from build123d import *

# Parameters (mm, degrees)
ESQUISSE1_R                  = 23.35
BOSS_EXTRU_1_DEPTH           = 5
ESQUISSE2_W                  = 37
ESQUISSE2_H                  = 8
ESQUISSE2_W_2                = 33.6
ESQUISSE2_H_2                = 14.6
ENL_V_MAT_EXTRU_4_DEPTH      = 3
ESQUISSE10_R                 = 23.35
BOSS_EXTRU_2_DEPTH           = 60
ENL_V_MAT_EXTRU_5_DEPTH      = 73.90709842
ENL_V_MAT_EXTRU_5_DEPTH_BACK = 73.90709842
ESQUISSE11_W                 = 20
ESQUISSE11_H                 = 45
ENL_V_MAT_EXTRU_6_DEPTH      = 73.90709842
ENL_V_MAT_EXTRU_6_DEPTH_BACK = 73.90709842
ESQUISSE12_W                 = 20
ESQUISSE12_H                 = 45
ESQUISSE13_W                 = 18.2
ESQUISSE13_H                 = 4.5
ESQUISSE13_W_2               = 16.2
ESQUISSE13_H_2               = 2.5
BOSS_EXTRU_4_DEPTH           = 50
ENL_V_MAT_EXTRU_7_DEPTH      = 65.151734193
ENL_V_MAT_EXTRU_7_DEPTH_BACK = 17
ESQUISSE16_W                 = 15
ESQUISSE16_H                 = 5
BOSS_EXTRU_5_DEPTH           = 20
BOSS_EXTRU_6_DEPTH           = 15
BOSS_EXTRU_7_START           = -5
ESQUISSE18_R                 = 1.5
BOSS_EXTRU_7_DEPTH           = 5
BOSS_EXTRU_8_DEPTH           = 12
BOSS_EXTRU_9_DEPTH           = 23


with BuildPart() as part:
    # Esquisse1 → Boss.-Extru.1 (new body)
    with BuildSketch(Plane(origin=(0, 0, 0), x_dir=(1, 0, 0), z_dir=(0, 1, 0))):
        with Locations(Location((0, 0, 0), (0, 0, 270))):
            Circle(ESQUISSE1_R)
    extrude(amount=BOSS_EXTRU_1_DEPTH)

    # Esquisse2 → Enlèv. mat.-Extru.4 (cut)
    with BuildSketch(Plane(origin=(0, 5, 0), x_dir=(1, 0, 0), z_dir=(0, 1, 0))):
        with Locations((0, 6)):
            Rectangle(ESQUISSE2_W, ESQUISSE2_H)
        with Locations((0, -6.3)):
            Rectangle(ESQUISSE2_W_2, ESQUISSE2_H_2)
    extrude(amount=-ENL_V_MAT_EXTRU_4_DEPTH, mode=Mode.SUBTRACT)

    # Esquisse10 → Boss.-Extru.2 (add)
    with BuildSketch(Plane(origin=(0, 5, 0), x_dir=(1, 0, 0), z_dir=(0, 1, 0))):
        with Locations(Location((0, 0, 0), (0, 0, 270))):
            Circle(ESQUISSE10_R)
        with BuildLine():
            ThreePointArc((-16.8, -13.175071157), (-6.969307713, 20.180467041), (21.35, 0))
            ThreePointArc((21.35, 0), (20.180467041, -6.969307713), (16.8, -13.175071157))
            Line((16.8, -13.175071157), (16.8, -13.6))
            Line((16.8, -13.6), (16.457900838, -13.6))
            ThreePointArc((16.457900838, -13.6), (0, -21.35), (-16.457900838, -13.6))
            Line((-16.457900838, -13.6), (-16.8, -13.6))
            Line((-16.8, -13.6), (-16.8, -13.175071157))
        make_face(mode=Mode.SUBTRACT)
    extrude(amount=BOSS_EXTRU_2_DEPTH)

    # Esquisse11 → Enlèv. mat.-Extru.5 (cut, two sides: drawn at the far end of the back side and taken through both)
    with BuildSketch(Plane.XY.offset(-ENL_V_MAT_EXTRU_5_DEPTH_BACK)):
        with Locations((0, 27.5)):
            Rectangle(ESQUISSE11_W, ESQUISSE11_H)
    extrude(amount=ENL_V_MAT_EXTRU_5_DEPTH + ENL_V_MAT_EXTRU_5_DEPTH_BACK, mode=Mode.SUBTRACT)

    # Esquisse12 → Enlèv. mat.-Extru.6 (cut, two sides: drawn at the far end of the back side and taken through both)
    with BuildSketch(Plane(origin=(0, 0, 0), x_dir=(0, 0, -1), z_dir=(1, 0, 0)).offset(-ENL_V_MAT_EXTRU_6_DEPTH_BACK)):
        with Locations((0, 27.5)):
            Rectangle(ESQUISSE12_W, ESQUISSE12_H)
    extrude(amount=ENL_V_MAT_EXTRU_6_DEPTH + ENL_V_MAT_EXTRU_6_DEPTH_BACK, mode=Mode.SUBTRACT)

    # Esquisse13 → Boss.-Extru.4 (add)
    # profile 1 of 3: a face of its own
    with BuildSketch(Plane(origin=(0, 5, 0), x_dir=(1, 0, 0), z_dir=(0, 1, 0))):
        with BuildLine():
            Line((17.8, 2), (-17.8, 2))
            Line((-17.8, 2), (-17.8, -11.789083934))
            ThreePointArc((-17.8, -11.789083934), (-17.31387421, -12.49208789), (-16.8, -13.175071157))
            Line((-16.8, -13.175071157), (-16.8, 1))
            Line((-16.8, 1), (16.8, 1))
            Line((16.8, 1), (16.8, -13.175071157))
            ThreePointArc((16.8, -13.175071157), (17.31387421, -12.49208789), (17.8, -11.789083934))
            Line((17.8, -11.789083934), (17.8, 2))
        make_face()
    # profile 2 of 3: a face of its own
    with BuildSketch(Plane(origin=(0, 5, 0), x_dir=(1, 0, 0), z_dir=(0, 1, 0))):
        with Locations((0, -15.85)):
            Rectangle(ESQUISSE13_W, ESQUISSE13_H)
        with Locations((0, -15.85)):
            Rectangle(ESQUISSE13_W_2, ESQUISSE13_H_2, mode=Mode.SUBTRACT)
    # profile 3 of 3: a face of its own
    with BuildSketch(Plane(origin=(0, 5, 0), x_dir=(1, 0, 0), z_dir=(0, 1, 0))):
        with Locations((0, -15.85)):
            Rectangle(ESQUISSE13_W_2, ESQUISSE13_H_2)
    extrude(amount=BOSS_EXTRU_4_DEPTH)

    # Esquisse15 → Enlèv. mat.-Extru.7 (cut, two sides: drawn at the far end of the back side and taken through both)
    with BuildSketch(Plane(origin=(0, 55, 0), x_dir=(1, 0, 0), z_dir=(0, 1, 0)).offset(-ENL_V_MAT_EXTRU_7_DEPTH_BACK)):
        Polygon((8.1, -14.6), (-8.1, -14.6), (-8.1, -17.1), (-6.1, -17.1), (-6.1, -18.1), (6.1, -18.1), (6.1, -17.1), (8.1, -17.1), align=None)
    extrude(amount=ENL_V_MAT_EXTRU_7_DEPTH + ENL_V_MAT_EXTRU_7_DEPTH_BACK, mode=Mode.SUBTRACT)

    # Esquisse16 → Boss.-Extru.5 (add)
    with BuildSketch(Plane(origin=(0, 5, 0), x_dir=(1, 0, 0), z_dir=(0, 1, 0))):
        with Locations((0, 15.5)):
            Rectangle(ESQUISSE16_W, ESQUISSE16_H)
    extrude(amount=BOSS_EXTRU_5_DEPTH)

    # Esquisse17 → Boss.-Extru.6 (add)
    with BuildSketch(Plane(origin=(0, 25, 0), x_dir=(1, 0, 0), z_dir=(0, 1, 0))):
        Polygon((7.5, 18), (-0.6, 18), (-0.6, 17), (5.6, 17), (5.6, 14), (-5.6, 14), (-5.6, 16.758406292), (-5.6, 18), (-7.5, 18), (-7.5, 13), (7.5, 13), align=None)
    extrude(amount=BOSS_EXTRU_6_DEPTH)

    # Esquisse18 → Boss.-Extru.7 (add)
    # profile 1 of 4: a face of its own
    with BuildSketch(Plane(origin=(0, 65, 0), x_dir=(1, 0, 0), z_dir=(0, 1, 0)).offset(BOSS_EXTRU_7_START)):
        with BuildLine():
            Line((-11.385882097, 13.385882097), (-11.385882097, 20.385882097))
            ThreePointArc((-11.385882097, 20.385882097), (-16.510943341, 16.510943341), (-20.385882097, 11.385882097))
            Line((-20.385882097, 11.385882097), (-13.385882097, 11.385882097))
            ThreePointArc((-13.385882097, 11.385882097), (-11.971668535, 11.971668535), (-11.385882097, 13.385882097))
        make_face()
        with Locations(Location((-13.385882097, 13.385882097, 0), (0, 0, 270))):
            Circle(ESQUISSE18_R, mode=Mode.SUBTRACT)
    # profile 2 of 4: a face of its own
    with BuildSketch(Plane(origin=(0, 65, 0), x_dir=(1, 0, 0), z_dir=(0, 1, 0)).offset(BOSS_EXTRU_7_START)):
        with BuildLine():
            ThreePointArc((20.385882097, 11.385882097), (16.510943341, 16.510943341), (11.385882097, 20.385882097))
            Line((11.385882097, 20.385882097), (11.385882097, 13.385882097))
            ThreePointArc((11.385882097, 13.385882097), (11.971668535, 11.971668535), (13.385882097, 11.385882097))
            Line((13.385882097, 11.385882097), (20.385882097, 11.385882097))
        make_face()
        with Locations(Location((13.385882097, 13.385882097, 0), (0, 0, 270))):
            Circle(ESQUISSE18_R, mode=Mode.SUBTRACT)
    # profile 3 of 4: a face of its own
    with BuildSketch(Plane(origin=(0, 65, 0), x_dir=(1, 0, 0), z_dir=(0, 1, 0)).offset(BOSS_EXTRU_7_START)):
        with BuildLine():
            Line((-13.385882097, -11.385882097), (-20.385882097, -11.385882097))
            ThreePointArc((-20.385882097, -11.385882097), (-16.510943341, -16.510943341), (-11.385882097, -20.385882097))
            Line((-11.385882097, -20.385882097), (-11.385882097, -13.385882097))
            ThreePointArc((-11.385882097, -13.385882097), (-11.971668535, -11.971668535), (-13.385882097, -11.385882097))
        make_face()
        with Locations(Location((-13.385882097, -13.385882097, 0), (0, 0, 270))):
            Circle(ESQUISSE18_R, mode=Mode.SUBTRACT)
    # profile 4 of 4: a face of its own
    with BuildSketch(Plane(origin=(0, 65, 0), x_dir=(1, 0, 0), z_dir=(0, 1, 0)).offset(BOSS_EXTRU_7_START)):
        with BuildLine():
            ThreePointArc((11.385882097, -20.385882097), (16.510943341, -16.510943341), (20.385882097, -11.385882097))
            Line((20.385882097, -11.385882097), (13.385882097, -11.385882097))
            ThreePointArc((13.385882097, -11.385882097), (11.971668535, -11.971668535), (11.385882097, -13.385882097))
            Line((11.385882097, -13.385882097), (11.385882097, -20.385882097))
        make_face()
        with Locations(Location((13.385882097, -13.385882097, 0), (0, 0, 270))):
            Circle(ESQUISSE18_R, mode=Mode.SUBTRACT)
    extrude(amount=BOSS_EXTRU_7_DEPTH)

    # Esquisse33 → Boss.-Extru.8 (add)
    with BuildSketch(Plane(origin=(0, 5, 0), x_dir=(1, 0, 0), z_dir=(0, 1, 0))):
        with BuildLine():
            Line((-19.5, 2), (-18.5, 2))
            Line((-18.5, 2), (-18.5, 10))
            Line((-18.5, 10), (18.5, 10))
            Line((18.5, 10), (18.5, 2))
            Line((18.5, 2), (19.5, 2))
            Line((19.5, 2), (19.5, 8.693244504))
            Line((19.5, 8.693244504), (19.5, 10))
            Line((19.5, 10), (18.863257937, 10))
            ThreePointArc((18.863257937, 10), (18.587432982, 10.503800986), (18.298155645, 11))
            Line((18.298155645, 11), (18.128988944, 11))
            Line((18.128988944, 11), (-18.298155645, 11))
            ThreePointArc((-18.298155645, 11), (-18.587432982, 10.503800986), (-18.863257937, 10))
            Line((-18.863257937, 10), (-19.5, 10))
            Line((-19.5, 10), (-19.5, 8.693244504))
            Line((-19.5, 8.693244504), (-19.5, 2))
        make_face()
    extrude(amount=BOSS_EXTRU_8_DEPTH)

    # Esquisse34 → Boss.-Extru.9 (add)
    with BuildSketch(Plane(origin=(0, 17, 0), x_dir=(1, 0, 0), z_dir=(0, 1, 0))):
        with BuildLine():
            Line((-18.5, 10), (18.5, 10))
            Line((18.5, 10), (18.5, 10.657039927))
            ThreePointArc((18.5, 10.657039927), (18.399876905, 10.828990252), (18.298155645, 11))
            Line((18.298155645, 11), (-18.298155645, 11))
            ThreePointArc((-18.298155645, 11), (-18.587432982, 10.503800986), (-18.863257937, 10))
            Line((-18.863257937, 10), (-19.5, 10))
            Line((-19.5, 10), (-19.5, 2))
            Line((-19.5, 2), (-18.5, 2))
            Line((-18.5, 2), (-18.5, 10))
        make_face()
    extrude(amount=BOSS_EXTRU_9_DEPTH)


solid = part.part
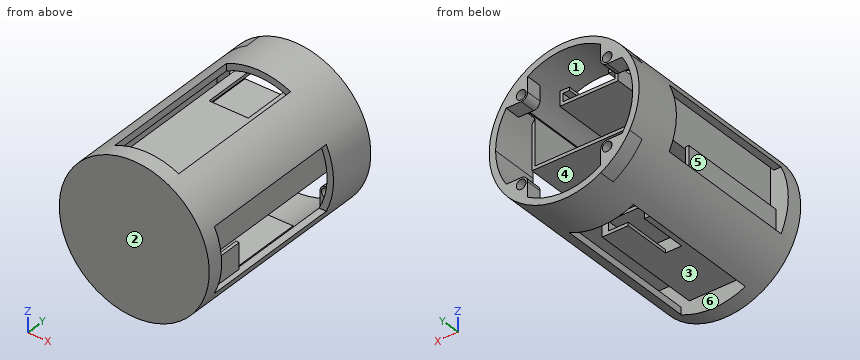
For this review, take the finished solid that the model builds, in its own axes (mm). Face numbers are marked on the shaded views. A direction names the side the tool comes from. Coordinates: 2 decimals unless noted, no trailing zeros. Write each loop counter-clockwise with the first axis right and the second up, starting at its lowest first coordinate (ties: lowest second). Pieces come first, ordered by that corner, then holes. Notation, with made-up numbers: (-35.75, 37.5) -> (4.25, 37.5) arc R9 ccw to (4.25, 46.5) -> close; hole circle Ø1 at (-8.5, 67). An arc over 180 degrees is marked (long way). Write each question's results on one line, items separated by ' | '. Start each with the question number.
1) For the marked faces 4, 5 and 6, list the 3-axis set-ups (+Z, -Z, +X, -X, +Y, -Y) from which the entire face can be reached by the end or side of a thin tool; tool diameter is ignored.
2) The part is to be moulded in two halves that separate along Z. For the marked faces 1, 2 and 3, say which applies: +Z half, -Z half, draft (parallel to the pull), parting line (faces both ways), or undercut.
3) Insertion check: pin 1 (12 mm diameter, centred on x = 1.5, y = 28.5, fed in from +Z); pin 2 (9 mm diameter, centred on y = 14, z = -5, fed in from +X); pin 3 (3 mm diameter, centred on x = 1, z = 17, fed in from +Y). Each pin has a flat end and moves straight along its axis. Give the tip position at first contact, or say it passes through.
4) Consider section B-B (y = 6.5). Give the number of separate pieces and of enclosed holes in the cut face, plus the area to 3 significant figures.
5) Wall thickness on L1, parallel to Z at x = 0, y = 35.5; L2, parallel to Y at x = -6.5, z = 21; L3, parallel to Z at x = 1, y = 53.5: over which ranges is each line inside the solid? List them lowest first. Write a range as [from, to].
6) Consider section A-A (y = 53.5). Write out the cut boundary in (x, z).
Geometry says:
1) face 4: +Y | face 5: -X | face 6: none
2) face 1: undercut | face 2: draft | face 3: -Z half
3) pin 1: z = 18.1 | pin 2: x = 19.5 | pin 3: y = 38
4) separate pieces: 4 | enclosed holes: 0 | area: 387 mm^2
5) L1: [-18, -17], [-14, -13], [-11, -10], [-2, -1], [13.6, 18.1] | L2: [0, 5], [50, 65] | L3: [-23.33, -21.33], [-2, -1], [13.6, 14.6], [21.33, 23.33]
6) outline: circle Ø46.7 at (0, 0); (-9.1, 13.6) -> (9.1, 13.6) -> (9.1, 18.1) -> (6.1, 18.1) -> (6.1, 17.1) -> (8.1, 17.1) -> (8.1, 14.6) -> (-8.1, 14.6) -> (-8.1, 17.1) -> (-6.1, 17.1) -> (-6.1, 18.1) -> (-9.1, 18.1) -> close; hole (-17.8, -2) -> (-17.8, 11.79) arc R21.35 ccw (long way) to (17.8, 11.79) -> (17.8, -2) -> close; hole (-16.8, -1) -> (16.8, -1) -> (16.8, 13.6) -> (16.46, 13.6) arc R21.35 ccw to (-16.46, 13.6) -> (-16.8, 13.6) -> close
